The model under review builds one solid part; all positions refer to its coordinate system, in mm. A direction names the side the tool comes from. Give positions to 0.01 mm unless a question says otherwise; leave off trailing zeros. Write each loop counter-clockwise with the first axis right and the second up, starting at its lowest first coordinate (ties: lowest second). Pieces come first, ordered by that corner, then holes. Notation, with made-up numbers: (-8, 33) -> (13, 33) arc R23 cw to (13, 66) -> close; hole circle Ø2 at (-7, -28). An arc over 180 degrees is marked (long way). Use CSV: the item, a comma, the result in double quotes.
```python
from build123d import *

# Parameters (mm, degrees)
CROQUIS1_W              = 50
CROQUIS1_H              = 50
SALIENTE_EXTRUIR1_DEPTH = 3
CROQUIS2_W              = 30
CROQUIS2_H              = 30
CROQUIS2_W_2            = 18
CROQUIS2_H_2            = 18
SALIENTE_EXTRUIR2_DEPTH = 30
CROQUIS3_R              = 2.813865728
CORTAR_EXTRUIR1_DEPTH   = 10
CROQUIS4_W              = 30
CROQUIS4_H              = 30
CROQUIS4_W_2            = 23.4
CROQUIS4_H_2            = 22.8
CORTAR_EXTRUIR2_DEPTH   = 15
REDONDEO1_R             = 2
CROQUIS5_W              = 18
CROQUIS5_H              = 18
CORTAR_EXTRUIR3_DEPTH   = 16
CROQUIS6_W              = 1
CROQUIS6_H              = 15.294109798
CORTAR_EXTRUIR4_DEPTH   = 37.7
CROQUIS7_W              = 1
CROQUIS7_H              = 15.234542974
CORTAR_EXTRUIR5_DEPTH   = 37.4


with BuildPart() as part:
    # Croquis1 → Saliente-Extruir1 (new body)
    with BuildSketch(Plane(origin=(0, 0, 0), x_dir=(1, 0, 0), z_dir=(0, 1, 0))):
        Rectangle(CROQUIS1_W, CROQUIS1_H)
    extrude(amount=SALIENTE_EXTRUIR1_DEPTH)

    # Croquis2 → Saliente-Extruir2 (add)
    with BuildSketch(Plane(origin=(0, 3, 0), x_dir=(1, 0, 0), z_dir=(0, 1, 0))):
        Rectangle(CROQUIS2_W, CROQUIS2_H)
        Rectangle(CROQUIS2_W_2, CROQUIS2_H_2, mode=Mode.SUBTRACT)
    extrude(amount=SALIENTE_EXTRUIR2_DEPTH)

    # Croquis3 → Cortar-Extruir1 (cut)
    with BuildSketch(Plane(origin=(0, 3, 0), x_dir=(1, 0, 0), z_dir=(0, 1, 0))):
        with Locations((15.405421421, -20)):
            Circle(CROQUIS3_R)
        with Locations((-15.676153635, -20)):
            Circle(CROQUIS3_R)
        with Locations((15.676153635, 20)):
            Circle(CROQUIS3_R)
        with Locations((-15.676153635, 20)):
            Circle(CROQUIS3_R)
    extrude(amount=-CORTAR_EXTRUIR1_DEPTH, mode=Mode.SUBTRACT)

    # Croquis4 → Cortar-Extruir2 (cut)
    with BuildSketch(Plane(origin=(0, 33, 0), x_dir=(1, 0, 0), z_dir=(0, 1, 0))):
        Rectangle(CROQUIS4_W, CROQUIS4_H)
        Rectangle(CROQUIS4_W_2, CROQUIS4_H_2, mode=Mode.SUBTRACT)
    extrude(amount=-CORTAR_EXTRUIR2_DEPTH, mode=Mode.SUBTRACT)

    # Redondeo1
    redondeo1_edges = [part.edges().sort_by_distance(p)[0] for p in [
        (-11.7, 33, 0),
        (-11.7, 25.5, -11.4),
        (0, 33, -11.4),
        (11.7, 25.5, -11.4),
        (11.7, 33, 0),
        (11.7, 25.5, 11.4),
        (0, 33, 11.4),
        (-11.7, 25.5, 11.4),
    ]]
    fillet(redondeo1_edges, radius=REDONDEO1_R)

    # Croquis5 → Cortar-Extruir3 (cut)
    with BuildSketch(Plane.XZ):
        Rectangle(CROQUIS5_W, CROQUIS5_H)
    extrude(amount=-CORTAR_EXTRUIR3_DEPTH, mode=Mode.SUBTRACT)

    # Croquis6 → Cortar-Extruir4 (cut, through all)
    with BuildSketch(Plane.ZY.offset(11.7)):
        with Locations((0, 25.647054899)):
            Rectangle(CROQUIS6_W, CROQUIS6_H)
    extrude(amount=-CORTAR_EXTRUIR4_DEPTH, mode=Mode.SUBTRACT)

    # Croquis7 → Cortar-Extruir5 (cut, through all)
    with BuildSketch(Plane.XY.offset(11.4)):
        with Locations((0, 25.617271487)):
            Rectangle(CROQUIS7_W, CROQUIS7_H)
    extrude(amount=-CORTAR_EXTRUIR5_DEPTH, mode=Mode.SUBTRACT)


solid = part.part
```
Q1. Consider section A-A (z = 20). Write out the cut boundary in (x, y), then the cut area to 3 significant figures.
Derived:
outline,"(-25, 0) -> (-18.49, 0) -> (-18.49, 3) -> (-25, 3) -> close; (-12.86, 0) -> (12.59, 0) -> (12.59, 3) -> (-12.86, 3) -> close; (18.22, 0) -> (25, 0) -> (25, 3) -> (18.22, 3) -> close"
area,"116 mm2"
Q2. Insertion check: pin 1 (4.5 mm diameter, centred on x = 4.5, y = 8.5, fed in from +Z); pin 2 (2.5 mm diameter, centred on y = 24.5, z = -11, fed in from +X); pin 3 (10 mm diameter, centred on y = 21.5, z = 3, fed in from +X). Each pin has a flat end and moves straight along its axis. Give the tip position at first contact, or say it passes through.
Derived:
pin 1,"stops at z = 15"
pin 2,"stops at x = 11.67"
pin 3,"stops at x = 15"
Q3. Consider section B-B (y = 4). Write out the cut boundary in (x, z), then the cut area to 3 significant figures.
Derived:
outline,"(-15, -15) -> (15, -15) -> (15, 15) -> (-15, 15) -> close; hole (-9, -9) -> (9, -9) -> (9, 9) -> (-9, 9) -> close"
area,"576 mm2"
Q4. Consider section D-D (y = 23.5). Write out the cut boundary in (x, z), then the cut area to 3 significant figures.
Derived:
outline,"(-11.7, -9.4) arc R2 ccw to (-9.7, -11.4) -> (-0.5, -11.4) -> (-0.5, -9) -> (-9, -9) -> (-9, -0.5) -> (-11.7, -0.5) -> close; (-11.7, 0.5) -> (-9, 0.5) -> (-9, 9) -> (-0.5, 9) -> (-0.5, 11.4) -> (-9.7, 11.4) arc R2 ccw to (-11.7, 9.4) -> close; (0.5, -11.4) -> (9.7, -11.4) arc R2 ccw to (11.7, -9.4) -> (11.7, -0.5) -> (9, -0.5) -> (9, -9) -> (0.5, -9) -> close; (0.5, 9) -> (9, 9) -> (9, 0.5) -> (11.7, 0.5) -> (11.7, 9.4) arc R2 ccw to (9.7, 11.4) -> (0.5, 11.4) -> close"
area,"196 mm2"
Q5. To check wall thickness, follow probe 1 along X at (y, z) = (1.05, 20); probe 2 along Z at (x, y) = (-0.5, 8.5); probe 3 along X at (y, z) = (1, -20). State the ranges of each line that lie inside material, in increasing order.
Derived:
probe 1,"x = -25 to -18.49, -12.86 to 12.59, 18.22 to 25"
probe 2,"z = -15 to -9, 9 to 15"
probe 3,"x = -25 to -18.49, -12.86 to 12.86, 18.49 to 25"
Q6. Consider section C-C (x = 5). Write out the cut boundary in (y, z), then the cut area to 3 significant figures.
Derived:
outline,"(0, -25) -> (3, -25) -> (3, -15) -> (18, -15) -> (18, -11.4) -> (31, -11.4) arc R2 ccw to (33, -9.4) -> (33, -9) -> (0, -9) -> close; (0, 9) -> (33, 9) -> (33, 9.4) arc R2 ccw to (31, 11.4) -> (18, 11.4) -> (18, 15) -> (3, 15) -> (3, 25) -> (0, 25) -> close"
area,"346 mm2"
Q7. The part is to be moulded in two halves that separate along X. For faces 4 (the flat face through (0, 10, 15)), 5 (the flat face through (25, 1, 0)), 6 (the cylindrical face through (-14.16, 1.52, -22.37)), say which applies: pulls with the +X half, pulls with the -X half, needs draft (parallel to the pull), parting line crosses it, or undercut.
Derived:
face 4,"needs draft"
face 5,"pulls with the +X half"
face 6,"undercut"
Q8. Machinability: for faces 1 (the flat face through (5, 25, 11.4)), 2 (the flat face through (-11.7, 25, -5)), 3 (the flat face through (10, 25, -0.5)), which of the approach directions +Z, -Z, +X, -X, +Y, -Y give a long, thin tool a straight path to every point of the face, cutting with its end or side? Answer none if there is none.
Derived:
face 1,"+Z, +X, -X, +Y"
face 2,"+Z, -Z, -X, +Y"
face 3,"+X, -X, +Y"
